Build history of the part. All positions in model axes, mm. Round coordinates to 2 decimals unless told otherwise and drop trailing zeros. Write each loop counter-clockwise with the first axis right and the second up, starting at its lowest first coordinate (ties: lowest second). Pieces come first, ordered by that corner, then holes. Notation, with made-up numbers: (-27, 15.5) - (-18, 15.5) arc R24 ccw to (-18, 28.5) - close; hole circle Ø3 at (0.25, -13.5). An arc over 180 degrees is marked (long way). Answer as a JSON object with one key per item and string values. Group by question number.
Item 1: Slice it at A-A, the plane x = 0. List the corners of the cut face in (y, z) (3 decimals).
Item 2: Slice it at B-B, the plane y = -44. List the corners of the cut face in (x, z) (3 decimals).
Item 3: Probe line 1 (Y direction, x = -79, z = 0.6); line 2 (Y direction, x = 0, z = 1.4) (3 decimals); line 3 (X direction, y = 84.5, z = 2.45) (3 decimals). List the from-to ranges inside material, lowest first. Write a range as from..to.
Item 4: Slice it at D-D, the plane x = 39.5. List the corners of the cut face in (y, z) (3 decimals), then the cut area to 3 significant figures.
Item 5: Flat gauge pins, fed straight in: pin 1 (1 mm diameter, centred on x = -109, z = 0.5, fed in from +Y); pin 2 (1.6 mm diameter, centred on y = -126, z = 2, fed in from -X); pin 3 (1.5 mm diameter, centred on x = 123, z = 2, fed in from +Y). Where does each tip first touch, or does it go through?
Item 6: Slice it at C-C, the plane y = 0. List the corners of the cut face in (x, z) (3 decimals).
Item 7: Two-plate mould, pull along Y, no slides. Class faces 1 (the flat face through (-3, -40, 3.175)), 2 (the cylindrical face through (-88.044, -150.805, 1.565)), 3 (the flat face through (-81.84, 65.58, 1.57)), 4 (the cylindrical face through (-41.98, -189.07, 1.57)): +Y half, -Y half, draft (parallel to the pull), parting line (faces both ways), or undercut.
from build123d import *

# Parameters (mm, degrees)
SKETCH1_R             = 193.675
SKETCH1_R_2           = 174.625
BOSS_EXTRUDE1_DEPTH   = 3.175
SKETCH1_R_3           = 34.925
SKETCH1_R_4           = 15.875
BOSS_EXTRUDE1_2_DEPTH = 3.175
BOSS_EXTRUDE2_START   = -3.175
SKETCH2_R             = 15.875
BOSS_EXTRUDE2_DEPTH   = 3.175


with BuildPart() as part:
    # Sketch1 → Boss-Extrude1 (new body)
    with BuildSketch(Plane.XY):
        Circle(SKETCH1_R)
        Circle(SKETCH1_R_2, mode=Mode.SUBTRACT)
    extrude(amount=BOSS_EXTRUDE1_DEPTH)



with BuildPart() as body_2:
    # Sketch1 → Boss-Extrude1 2 (new body)
    with BuildSketch(Plane.XY):
        Circle(SKETCH1_R_3)
        Circle(SKETCH1_R_4, mode=Mode.SUBTRACT)
    extrude(amount=BOSS_EXTRUDE1_2_DEPTH)


with BuildPart() as part_1:
    add(part.part)

    add(body_2.part)  # Boss-Extrude2 merges body 2
    # Sketch2 → Boss-Extrude2 (add)
    with BuildSketch(Plane.XY.offset(3.175).offset(BOSS_EXTRUDE2_START)):
        with BuildLine():
            Line((15.875, 49.493351826), (15.875, 159.383735055))
            ThreePointArc((15.875, 159.383735055), (20.425550361, 169.124190413), (30.816176471, 171.884420157))
            ThreePointArc((30.816176471, 171.884420157), (0, 174.625), (-30.816176471, 171.884420157))
            ThreePointArc((-30.816176471, 171.884420157), (-20.425550361, 169.124190413), (-15.875, 159.383735055))
            Line((-15.875, 159.383735055), (-15.875, 49.493351826))
            ThreePointArc((-15.875, 49.493351826), (-22.225, 38.494829198), (-34.925, 38.494829198))
            Line((-34.925, 38.494829198), (-130.092863507, 93.440020812))
            ThreePointArc((-130.092863507, 93.440020812), (-136.253070112, 102.251140706), (-133.448186135, 112.62980175))
            ThreePointArc((-133.448186135, 112.62980175), (-151.229686136, 87.3125), (-164.264362606, 59.254618408))
            ThreePointArc((-164.264362606, 59.254618408), (-156.678620473, 66.873049707), (-145.967863507, 65.943714242))
            Line((-145.967863507, 65.943714242), (-50.8, 10.998522628))
            ThreePointArc((-50.8, 10.998522628), (-44.45, 0), (-50.8, -10.998522628))
            Line((-50.8, -10.998522628), (-145.967863507, -65.943714242))
            ThreePointArc((-145.967863507, -65.943714242), (-156.678620473, -66.873049707), (-164.264362606, -59.254618408))
            ThreePointArc((-164.264362606, -59.254618408), (-151.229686136, -87.3125), (-133.448186135, -112.62980175))
            ThreePointArc((-133.448186135, -112.62980175), (-136.253070112, -102.251140706), (-130.092863507, -93.440020812))
            Line((-130.092863507, -93.440020812), (-34.925, -38.494829198))
            ThreePointArc((-34.925, -38.494829198), (-22.225, -38.494829198), (-15.875, -49.493351826))
            Line((-15.875, -49.493351826), (-15.875, -159.383735055))
            ThreePointArc((-15.875, -159.383735055), (-20.425550361, -169.124190413), (-30.816176471, -171.884420157))
            ThreePointArc((-30.816176471, -171.884420157), (0, -174.625), (30.816176471, -171.884420157))
            ThreePointArc((30.816176471, -171.884420157), (20.425550361, -169.124190413), (15.875, -159.383735055))
            Line((15.875, -159.383735055), (15.875, -49.493351826))
            ThreePointArc((15.875, -49.493351826), (22.225, -38.494829198), (34.925, -38.494829198))
            Line((34.925, -38.494829198), (130.092863507, -93.440020812))
            ThreePointArc((130.092863507, -93.440020812), (136.253070112, -102.251140706), (133.448186135, -112.62980175))
            ThreePointArc((133.448186135, -112.62980175), (151.229686136, -87.3125), (164.264362606, -59.254618408))
            ThreePointArc((164.264362606, -59.254618408), (156.678620473, -66.873049707), (145.967863507, -65.943714242))
            Line((145.967863507, -65.943714242), (50.8, -10.998522628))
            ThreePointArc((50.8, -10.998522628), (44.45, 0), (50.8, 10.998522628))
            Line((50.8, 10.998522628), (145.967863507, 65.943714242))
            ThreePointArc((145.967863507, 65.943714242), (156.678620473, 66.873049707), (164.264362606, 59.254618408))
            ThreePointArc((164.264362606, 59.254618408), (151.229686136, 87.3125), (133.448186135, 112.62980175))
            ThreePointArc((133.448186135, 112.62980175), (136.253070112, 102.251140706), (130.092863507, 93.440020812))
            Line((130.092863507, 93.440020812), (34.925, 38.494829198))
            ThreePointArc((34.925, 38.494829198), (22.225, 38.494829198), (15.875, 49.493351826))
        make_face()
        Circle(SKETCH2_R, mode=Mode.SUBTRACT)
    extrude(amount=BOSS_EXTRUDE2_DEPTH)


solid = part_1.part
Geometry says:
{
 "1": {"outline": "(-193.675, 0) - (-15.875, 0) - (-15.875, 3.175) - (-193.675, 3.175) - close; (15.875, 0) - (193.675, 0) - (193.675, 3.175) - (15.875, 3.175) - close"},
 "2": {"outline": "(-188.611, 0) - (-168.991, 0) - (-168.991, 3.175) - (-188.611, 3.175) - close; (-107.96, 0) - (-44.46, 0) - (-44.46, 3.175) - (-107.96, 3.175) - close; (-17.125, 0) - (17.125, 0) - (17.125, 3.175) - (-17.125, 3.175) - close; (44.46, 0) - (107.96, 0) - (107.96, 3.175) - (44.46, 3.175) - close; (168.991, 0) - (188.611, 0) - (188.611, 3.175) - (168.991, 3.175) - close"},
 "3": {"line 1": "y = -176.83..-155.73, -63.94..-27.28, 27.28..63.94, 155.73..176.83", "line 2": "y = -193.675..-15.875, 15.875..193.675", "line 3": "x = -174.269..-114.608, -15.875..15.875, 114.608..174.269"},
 "4": {"outline": "(-189.604, 0) - (-170.099, 0) - (-170.099, 3.175) - (-189.604, 3.175) - close; (-41.136, 0) - (41.136, 0) - (41.136, 3.175) - (-41.136, 3.175) - close; (170.099, 0) - (189.604, 0) - (189.604, 3.175) - (170.099, 3.175) - close", "area": "385 mm^2"},
 "5": {"pin 1": "stops at y = 160.43", "pin 2": "stops at x = -147.77", "pin 3": "stops at y = 150.22"},
 "6": {"outline": "(-193.675, 0) - (-174.625, 0) - (-174.625, 3.175) - (-193.675, 3.175) - close; (-44.45, 0) - (-15.875, 0) - (-15.875, 3.175) - (-44.45, 3.175) - close; (15.875, 0) - (44.45, 0) - (44.45, 3.175) - (15.875, 3.175) - close; (174.625, 0) - (193.675, 0) - (193.675, 3.175) - (174.625, 3.175) - close"},
 "7": {"face 1": "draft", "face 2": "undercut", "face 3": "undercut", "face 4": "parting line"}
}
